from build123d import *

# Parameters (mm, degrees)
F0_W      = 10
F0_H      = 10
F7_DEPTH  = 10
F8_DEPTH  = 4.473135955
F9_DEPTH  = 4.473135955
F12_W     = 19.2976649851
F12_H     = 18.8721097074
F13_DEPTH = 4.473135955
F14_W     = 48.2514444739
F14_H     = 43.6994209886
F15_DEPTH = 4.473135955


with BuildPart() as f7:
    # F0 (on Top) → F7 (new body)
    with BuildSketch(Plane.XY):
        Rectangle(F0_W, F0_H)
    extrude(amount=F7_DEPTH)

    # F4 (on 3pt) → F8 (cut, through all)
    with BuildSketch(Plane(origin=(4, 0, 2), x_dir=(0, 1, 0), z_dir=(0.894427191, 0, 0.4472135955))):
        Polygon((0, 8.94427191), (-5, -2.2360679775), (5, -2.2360679775), align=None)
    extrude(amount=F8_DEPTH, mode=Mode.SUBTRACT)

    # F6 (on 3pt) → F9 (cut, through all)
    with BuildSketch(Plane(origin=(-4, 0, 2), x_dir=(0, 1, 0), z_dir=(0.894427191, 0, -0.4472135955))):
        Polygon((-5, -2.2360679775), (5, -2.2360679775), (0, 8.94427191), align=None)
    extrude(amount=-F9_DEPTH, mode=Mode.SUBTRACT)

    # F12 (on 3pt) → F13 (cut, through all)
    with BuildSketch(Plane(origin=(0, -4, 2), x_dir=(-1, 0, 0), z_dir=(0, 0.894427191, -0.4472135955))):
        with Locations((0.6115389988, 1.8165449146)):
            Rectangle(F12_W, F12_H)
    extrude(amount=-F13_DEPTH, mode=Mode.SUBTRACT)

    # F14 (on 3pt) → F15 (cut, through all)
    with BuildSketch(Plane(origin=(0, 4, 2), x_dir=(-1, 0, 0), z_dir=(0, 0.894427191, 0.4472135955))):
        with Locations((-1.8208147958, 2.8563160449)):
            Rectangle(F14_W, F14_H)
    extrude(amount=F15_DEPTH, mode=Mode.SUBTRACT)


solid = f7.part
For this review, take the finished solid that the model builds, in its own axes (mm). Round coordinates to 2 decimals unless told otherwise and drop trailing zeros. Write each loop counter-clockwise with the first axis right and the second up, starting at its lowest first coordinate (ties: lowest second). Pieces come first, ordered by that corner, then holes. Notation, with made-up numbers: M 65,-32.75 L 103,-32.75 A13 ccw 103,-18.75 Z; hole C 28.5,75.25 d11. An arc over 180 degrees is marked long. Write item = value, one per line. Start each with the question number.
(1) Clearance check with flat-ended pins moving along their axes: pin 1 Ø1 at (x, z) = (0.5, 4) entering from +Y; pin 2 Ø1.5 at (x, z) = (-3.5, 5) entering from -Y; pin 3 Ø1.5 at (x, z) = (0.5, 7) entering from -Y (3 decimals). State where each tip first meets the part, or that it passes through.
(2) We need section B-B (y = -3.5). Give the boundary of the cut face in (x, z).
(3) We need section A-A (z = 1.5). Give the boundary of the cut face in (x, y), then the cut area to 4 significant figures.
(4) For line 1 along Z through (x, y) = (-2.5, 1.75); line 2 along Z through (x, y) = (-3.25, -0.25); line 3 along X through (y, z) = (1, 4), list the stretches that pass through material, from the lowest coordinate up.
Results found:
q1.pin_1 = 3.25
q1.pin_2 = through
q1.pin_3 = -1.875
q2.outline = M -5,0 L 5,0 L 3.5,3 L -3.5,3 Z
q3.outline = M -4.25,-4.25 L 4.25,-4.25 L 4.25,4.25 L -4.25,4.25 Z
q3.area = 72.25 mm²
q4.line_1 = 0 to 5
q4.line_2 = 0 to 3.5
q4.line_3 = -3 to 3
